from build123d import *

# Parameters (mm, degrees)
SKETCH1_W              = 176
SKETCH1_H              = 350
BOSS_EXTRUDE1_DEPTH    = 3
F_5_0MM_DOWEL_HOLE1_D  = 5
F_12_0MM_DOWEL_HOLE1_D = 12


with BuildPart() as part:
    # Sketch1 → Boss-Extrude1 (new body)
    with BuildSketch(Plane(origin=(0, 0, 0), x_dir=(1, 0, 0), z_dir=(0, 1, 0))):
        with Locations((88, 175)):
            Rectangle(SKETCH1_W, SKETCH1_H)
    extrude(amount=BOSS_EXTRUDE1_DEPTH)

    # Ø5.0mm Dowel Hole1 (through all)
    with Locations(Plane(origin=(0, 0, 0), x_dir=(-1, 0, 0), z_dir=(0, -1, 0))):
        with Locations((-88.016913139, 250.06), (-88.016913139, 200.06)):
            Hole(F_5_0MM_DOWEL_HOLE1_D / 2)

    # Ø12.0mm Dowel Hole1 (through all)
    with Locations(Plane(origin=(0, 0, 0), x_dir=(-1, 0, 0), z_dir=(0, -1, 0))):
        with Locations((-88, 290)):
            Hole(F_12_0MM_DOWEL_HOLE1_D / 2)


solid = part.part
Check sheet for the modelled part. Datum: model origin and axes. Units: mm. Round coordinates to 2 decimals unless told otherwise and drop trailing zeros. Loops run counter-clockwise (first coordinate to the right, second up) from the corner with the lowest first, then second, coordinate; pieces in that order, holes last.
1. Mould release check, pull along Z, two halves, no side actions. Record for faces 1 (the flat face through (87, 3, -177)), 2 (the cylindrical face through (87.22, 1.52, -295.95)): released by +Z, released by -Z, zero draft, split by the parting line, or undercut.
2. Sectioned sample at A-A on z = -290. Record the boundary of the cut face in (x, y), and give its area (3 significant figures).
3. Scan lines: probe 1 along Z at (x, y) = (88, 1.4); probe 2 along X at (y, z) = (2.1, -200.06); probe 3 along X at (y, z) = (1.1, -292.5). Record each from-to range of solid material in increasing order.
Recorded:
1. face 1: zero draft
1. face 2: undercut
2. outline: (0, 0) - (82, 0) - (82, 3) - (0, 3) - close; (94, 0) - (176, 0) - (176, 3) - (94, 3) - close
2. area: 492 mm2
3. probe 1: z = -350 to -296, -284 to -252.56, -247.56 to -202.56, -197.56 to 0
3. probe 2: x = 0 to 85.52, 90.52 to 176
3. probe 3: x = 0 to 82.55, 93.45 to 176
